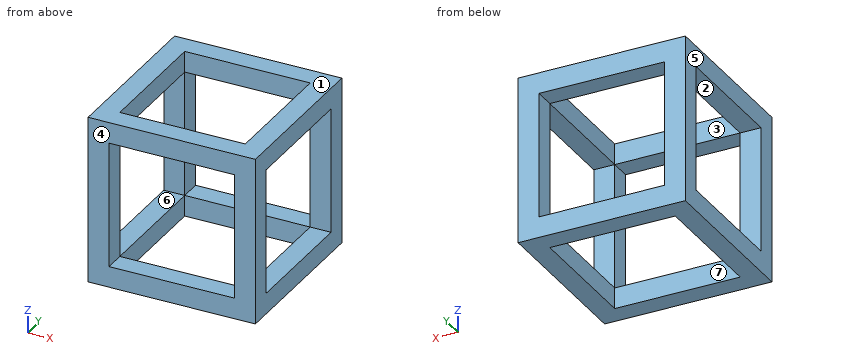
from build123d import *

# Parameters (mm, degrees)
F0_W      = 101.6
F0_H      = 101.6
F1_DEPTH  = 101.6
F2_W      = 76.2
F2_H      = 76.2
F3_DEPTH  = 76.2
F3_FACE_W = 76.2
F3_FACE_H = 76.2
F4_DEPTH  = 25.4
F5_W      = 76.2
F5_H      = 76.2
F6_DEPTH  = 101.6
F7_W      = 76.2
F7_H      = 76.2
F8_DEPTH  = 101.6


with BuildPart() as f1:
    # F0 (on Front) → F1 (new body)
    with BuildSketch(Plane.XZ):
        with Locations((-4.952999, 18.993384)):
            Rectangle(F0_W, F0_H)
    extrude(amount=-F1_DEPTH)

    # F2 (on face) → F3 (cut)
    with BuildSketch(Plane.XY.offset(69.793384)):
        with Locations((-4.952999, 50.8)):
            Rectangle(F2_W, F2_H)
    extrude(amount=-F3_DEPTH, mode=Mode.SUBTRACT)

    # F3_face (on face) → F4 (cut)
    with BuildSketch(Plane(origin=(-4.952999, 50.8, -6.406616), x_dir=(1, 0, 0), z_dir=(0, 0, 1))):
        Rectangle(F3_FACE_W, F3_FACE_H)
    extrude(amount=-F4_DEPTH, mode=Mode.SUBTRACT)

    # F5 (on face) → F6 (cut)
    with BuildSketch(Plane(origin=(0, 101.6, 0), x_dir=(-1, 0, 0), z_dir=(0, 1, 0))):
        with Locations((4.952999, 18.993384)):
            Rectangle(F5_W, F5_H)
    extrude(amount=-F6_DEPTH, mode=Mode.SUBTRACT)

    # F7 (on face) → F8 (cut)
    with BuildSketch(Plane.YZ.offset(45.847001)):
        with Locations((50.8, 18.993384)):
            Rectangle(F7_W, F7_H)
    extrude(amount=-F8_DEPTH, mode=Mode.SUBTRACT)


solid = f1.part
Build history of the part. All positions in model axes, mm. Face numbers are marked on the shaded views. A direction names the side the tool comes from. Round coordinates to 2 decimals unless told otherwise and drop trailing zeros. Write each loop counter-clockwise with the first axis right and the second up, starting at its lowest first coordinate (ties: lowest second). Pieces come first, ordered by that corner, then holes. Notation, with made-up numbers: M 67.25,-20 L 87.25,-20 A31 cw 87.25,13 Z; hole C 37,-2 d11. An arc over 180 degrees is marked long. Use CSV: the item, a comma, the result in double quotes.
1. Saw through at C-C (y = 92). Give the cut face in (x, z), plus the area to 3 significant figures.
Reply:
outline,"M -55.75,-31.81 L 45.85,-31.81 L 45.85,69.79 L -55.75,69.79 Z; hole M -43.05,-19.11 L 33.15,-19.11 L 33.15,57.09 L -43.05,57.09 Z"
area,"4,520 mm²"
2. Tool access for the marked faces 1, 2 and 3: list every direction of +Z, -Z, +X, -X, +Y, -Y with a clear straight run to the whole face (end or side of a thin tool).
Reply:
face 1,"+Z, +X, -X, +Y, -Y"
face 2,"+X, -X"
face 3,"+Z, -Z"
3. Wall check: probe 1 along Y at (x, z) = (-20.5, 62); probe 2 along Z at (x, y) = (-22.5, 92); probe 3 along X at (y, z) = (8, 52). Give the ranges that are in metal, low to high. Write a range as from..to.
Reply:
probe 1,"y = 0..12.7, 88.9..101.6"
probe 2,"z = -31.81..-19.11, 57.09..69.79"
probe 3,"x = -55.75..-43.05, 33.15..45.85"
4. Saw through at A-A (z = 54). Give the cut face in (x, y), plus the area to 3 significant figures.
Reply:
outline,"M -55.75,0 L -43.05,0 L -43.05,12.7 L -55.75,12.7 Z; M -55.75,88.9 L -43.05,88.9 L -43.05,101.6 L -55.75,101.6 Z; M 33.15,0 L 45.85,0 L 45.85,12.7 L 33.15,12.7 Z; M 33.15,88.9 L 45.85,88.9 L 45.85,101.6 L 33.15,101.6 Z"
area,"645 mm²"
5. Saw through at D-D (x = 39.5). Give the cut face in (y, z).
Reply:
outline,"M 0,-31.81 L 101.6,-31.81 L 101.6,69.79 L 0,69.79 Z; hole M 12.7,-19.11 L 88.9,-19.11 L 88.9,57.09 L 12.7,57.09 Z"
6. Saw through at B-B (x = 18). Give the cut face in (y, z).
Reply:
outline,"M 0,-31.81 L 12.7,-31.81 L 12.7,-19.11 L 0,-19.11 Z; M 0,57.09 L 12.7,57.09 L 12.7,69.79 L 0,69.79 Z; M 88.9,-31.81 L 101.6,-31.81 L 101.6,-19.11 L 88.9,-19.11 Z; M 88.9,57.09 L 101.6,57.09 L 101.6,69.79 L 88.9,69.79 Z"
7. Two-plate mould, pull along Y, no slides. Class the marked faces 4, 5, 6 and 7: +Y half, -Y half, draft (parallel to the pull), parting line (faces both ways), or undercut.
Reply:
face 4,"-Y half"
face 5,"draft"
face 6,"undercut"
face 7,"undercut"
